Autodesk Inventor part; units mm, degrees
ref_plane "Work Plane1" through (13.2035, 0, 0) normal (0, 0, 1) x (-1, 0, 0)
ref_plane "YZ Plane" through (0, 0, 0) normal (1, 0, 0) x (0, 1, 0)
ref_plane "XZ Plane" through (0, 0, 0) normal (0, 1, 0) x (-1, 0, 0)
sketch "Sketch1" plane through (0, 0, 0) normal (1, 0, 0) x (0, 1, 0)
  line L0 (2.3094, -4) -> (-2.3094, -4)
  line L1 (-2.3094, -4) -> (-4.6188, 0)
  line L2 (-4.6188, 0) -> (-2.3094, 4)
  line L3 (-2.3094, 4) -> (2.3094, 4)
  line L4 (2.3094, 4) -> (4.6188, 0)
  line L5 (4.6188, 0) -> (2.3094, -4)
  point P0 (0, 0)
  point P1 (0, 0)
  dimension "d0" = 9.2376
extrude "Body" add sketch "Sketch1" along normal blind 3.2
sketch "Sketch2" plane through (3.2, 0, 0) normal (1, 0, 0) x (0, 0, -1)
  circle A0 centre (0, 0) radius 3.45
  dimension "d7" = 6.9
extrude "Ring" add sketch "Sketch2" along normal blind 1.8
sketch "Sketch3" plane through (0, 0, 0) normal (0, 0, 1) x (1, 0, 0)
  line L0 (0, 2.3094) -> (0, 4.6188)
  line L1 (0, 4.6188) -> (3.2, 4.6188)
  line L2 (3.2, 2.3094) -> (3.2, 4.6188)
  line L3 (-0.64, 0) -> (3.84, 0)
  line L4 (0, 3.45) -> (0.6748, 4.6188)
  line L5 (2.5252, 4.6188) -> (3.2, 3.45)
  dimension "d3" = 30
  dimension "d4" = 30
  dimension "d5" = 6.9
  dimension "d6" = 6.9
revolve "Chamfer1" cut sketch "Sketch3" angle 360 about axis through (-10, 0, 0) along (1, 0, 0)
sketch "Sketch4" plane through (0, 0, 0) normal (-1, 0, 0) x (0, 0, 1)
  line L0 (0, -6.4663) -> (0, 6.4663)
  line L1 (-5.6, 0) -> (5.6, 0)
  point P0 (0, 0)
hole "Thread" at (0, 0, 0) direction (1, 0, 0) diameter 4.134 end through all
chamfer "Chamfer2" distance 0.433 angle 30 1 edges at (0, 0, -2.067) measured on face at (0, 2.9506, -0.3583)
chamfer "Chamfer3" distance 0.433 angle 30 1 edges at (5, 0, -2.067) measured on face at (5, -0.4401, -2.9356)
ref_plane "Work Plane1" through (13.2035, 0, 0) normal (0, 0, 1) x (-1, 0, 0)
equation "\"d0\" = 1.1547 * SW"
equation "\"d1\" = KOH1"
equation "\"d7\" = SD2"
equation "\"d8\" = KOH - KOH1"
equation "\"d3\" = ANG1"
equation "\"d4\" = ANG2"
equation "\"d5\" = SW0"
equation "\"d6\" = SW01"
equation "\"d10\" = -0.5 * GD1 + 0.5 * NND"
equation "\"d46\" = -0.5 * GD1 + 0.5 * NND"
equation "\"d12\" = -0.5 * GD1 + 0.5 * NND"
equation "\"d47\" = -0.5 * GD1 + 0.5 * NND"
equation "\"ANG1\" = 30deg"
equation "\"ANG2\" = 30deg"
equation "\"NND\" = 5"
equation "\"KOH1\" = 3.2"
equation "\"KOH\" = 5"
equation "\"SW\" = 8"
equation "\"SW0\" = 6.9"
equation "\"SW01\" = SW0"
equation "\"SD2\" = SW0"
equation "\"GUL\" = 0.541266 * PTC"
equation "\"THREADDIA\" = 5"
equation "\"TOA\" = 30deg"
equation "\"PTC\" = 0.8"
equation "\"GAL\" = 0.541266 * PTC"
equation "\"E0\" = 1.155 * SW"
properties part number "DIN 985 - M5" material "Steel, Mild"
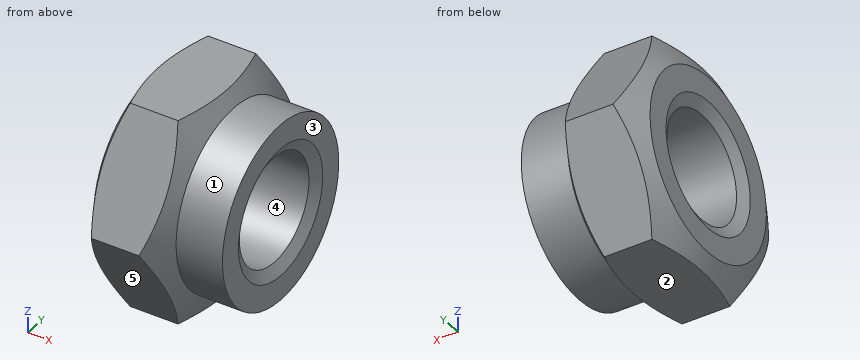
Input: part model. Units: mm. Frame: model coordinates. Face numbers are marked on the shaded views. A direction names the side the tool comes from. Round coordinates to 2 decimals unless told otherwise and drop trailing zeros. Loops run counter-clockwise (first coordinate to the right, second up) from the corner with the lowest first, then second, coordinate; pieces in that order, holes last. Notation, with made-up numbers: (84, 36) - (137, 36) arc R26 cw to (137, 75) - close; hole circle Ø8 at (48.5, 73). An arc over 180 degrees is marked (long way). One line per item, written item: value. Start each with the question number.
(1) Access query for the marked faces 1 and 2. Directions: +Z, -Z, +X, -X, +Y, -Y. A direction counts if a zero-diameter tool reaches every point of the face in a straight line with its end or side. Return the directions, or none.
(2) Section A-A, the plane y = 0. Return loops of the section in (x, z), plus the area to 3 significant figures.
(3) Contact query for flat-ended pins moving along their axis: P1, Ø1.5, axis at x = 2.5, z = -3, coming from the +Y side; P2, Ø3, axis at x = 1.5, z = 3, coming from the +Y side. Output: stop coordinate, or through.
(4) Draft query along Z for the marked faces 3, 4 and 5. Return one class per face: +Z half, -Z half, draft (parallel to the pull), parting line (faces both ways), or undercut.
(5) Ray query, line 1 (Y direction, x = 3.85, z = 0); line 2 (Z direction, x = 2.4, y = 0). Return the intervals inside material, ascending. Write a range as [from, to].
Results below:
1. face 1: +X
1. face 2: -Z, +X, -X, +Y, -Y
2. outline: (0, -3.45) - (0.32, -4) - (2.88, -4) - (3.2, -3.45) - (5, -3.45) - (5, -2.5) - (4.75, -2.07) - (0.25, -2.07) - (0, -2.5) - close; (0, 2.5) - (0.25, 2.07) - (4.75, 2.07) - (5, 2.5) - (5, 3.45) - (3.2, 3.45) - (2.88, 4) - (0.32, 4) - (0, 3.45) - close
2. area: 16.8 mm^2
3. P1: y = 3.32
3. P2: y = 3.75
4. face 3: draft
4. face 4: undercut
4. face 5: -Z half
5. line 1: [-3.45, -2.07], [2.07, 3.45]
5. line 2: [-4, -2.07], [2.07, 4]
